```python
from build123d import *

# Parameters (mm, degrees)
SKETCH1_W           = 3.375
SKETCH1_H           = 1
CUT_EXTRUDE1_DEPTH  = 17.505188578
CIRPATTERN1_COUNT   = 3
SKETCH5_R           = 0.4
BOSS_EXTRUDE1_DEPTH = 2.5


with BuildPart() as part:
    # Sketch1 → Revolve1 (revolve)
    with BuildSketch(Plane(origin=(0, 0, 0), x_dir=(0, 0, -1), z_dir=(1, 0, 0)), mode=Mode.PRIVATE) as revolve1_sk:
        with Locations((1.6875, 15.3)):
            Rectangle(SKETCH1_W, SKETCH1_H)
    revolve(revolve1_sk.sketch.rotate(Axis((0, 33.37320456, 0), (0, -1, 0)), 180), axis=Axis((0, 33.37320456, 0), (0, -1, 0)))

    # Sketch2 → Cut-Extrude1 (cut, through all)
    with BuildSketch(Plane(origin=(0, 0, 0), x_dir=(0, 0, -1), z_dir=(1, 0, 0))):
        with BuildLine():
            Line((-0.5, 15.8), (0.5, 15.8))
            ThreePointArc((0.5, 15.8), (0.321027237, 15.781039562), (0.15, 15.725))
            Line((0.15, 15.725), (0.15, 15.65))
            Line((0.15, 15.65), (-0.15, 15.65))
            Line((-0.15, 15.65), (-0.15, 15.725))
            ThreePointArc((-0.15, 15.725), (-0.321027237, 15.781039562), (-0.5, 15.8))
        make_face()
    cut_extrude1 = extrude(amount=-CUT_EXTRUDE1_DEPTH, mode=Mode.SUBTRACT)

    # CirPattern1: Cut-Extrude1 ×3 about axis
    cirpattern1_axis = Axis((0, 0, 0), (0, 1, 0))
    for i in range(1, CIRPATTERN1_COUNT):
        add(cut_extrude1.rotate(cirpattern1_axis, i * 360 / CIRPATTERN1_COUNT), mode=Mode.SUBTRACT)

    # Sketch1_3 → Revolve2 (revolve)
    with BuildSketch(Plane(origin=(0, 0, 0), x_dir=(0, 0, -1), z_dir=(1, 0, 0)), mode=Mode.PRIVATE) as revolve2_sk:
        with BuildLine():
            Line((3.375, 15.9), (3.375, 15.8))
            Line((3.375, 15.8), (3.375, 14.8))
            Line((3.375, 14.8), (0, 14.8))
            Line((0, 14.8), (0, 0))
            Line((0, 0), (4, 0))
            Line((4, 0), (4, -0.1))
            Line((4, -0.1), (4.15, -0.1))
            ThreePointArc((4.15, -0.1), (4.857106781, 0.192893219), (5.15, 0.9))
            Line((5.15, 0.9), (5.15, 1.95))
            ThreePointArc((5.15, 1.95), (5.092538314, 2.341511494), (4.925, 2.7))
            ThreePointArc((4.925, 2.7), (4.7, 3.45), (4.925, 4.2))
            ThreePointArc((4.925, 4.2), (5.092538314, 4.558488506), (5.15, 4.95))
            Line((5.15, 4.95), (5.15, 14.9))
            ThreePointArc((5.15, 14.9), (4.857106781, 15.607106781), (4.15, 15.9))
            Line((4.15, 15.9), (3.375, 15.9))
        make_face()
    revolve(revolve2_sk.sketch.rotate(Axis((0, 33.37320456, 0), (0, -1, 0)), 180), axis=Axis((0, 33.37320456, 0), (0, -1, 0)))

    # Sketch5 → Boss-Extrude1 (add)
    with BuildSketch(Plane.XZ):
        with Locations(Location((0, 2.5, 0), (0, 0, 270))):
            Circle(SKETCH5_R)
        with Locations(Location((0, -2.5, 0), (0, 0, 90))):
            Circle(SKETCH5_R)
    extrude(amount=BOSS_EXTRUDE1_DEPTH)


solid = part.part
```
Geometry check sheet. Reference: the model listing, model coordinates, mm. A direction names the side the tool comes from. Coordinates: 2 decimals unless noted, no trailing zeros. Order: outer loops, then holes, each group sorted by start corner. A loop starts at its lowest first (then second) coordinate and runs counter-clockwise, first axis right, second up.
Item 1: Scan lines: line 1 along Y through (x, z) = (0, -1.5); line 2 along Y through (x, z) = (0.75, 1.5); line 3 along Y through (x, z) = (-4.5, 2). Record each from-to range of solid material in increasing order.
Item 2: Depth check by flat-ended pin: pin 1 (1.5 mm diameter, centred on x = 1.5, y = 1.5, fed in from -Z); pin 2 (4 mm diameter, centred on y = 0.5, z = -4, fed in from -X); pin 3 (2.5 mm diameter, centred on x = -1.5, z = 1, fed in from -Y). Enter the tip coordinate at first touch or a pass-through.
Item 3: Tool access check on faces 1 (the flat face through (0, 0, 0)), 2 (the flat face through (0, 15.65, 0)), 3 (the flat face through (2, 15.9, 3)). Record the directions out of +Z, -Z, +X, -X, +Y, -Y that give a thin tool (end or side, any length) a straight path to the whole face; none if there is none.
Item 4: Section check A-A (y = 11.5). Enter the section's corners in (x, z).
Check sheet entries:
1. line 1: y = 0 to 15.8
1. line 2: y = 0 to 15.65
1. line 3: y = 0.27 to 2.7, 4.2 to 15.53
2. pin 1: stops at z = -5.1
2. pin 2: stops at x = -4.73
2. pin 3: stops at y = 0
3. face 1: -Y
3. face 2: +Y
3. face 3: +Z, -Z, +X, -X, +Y
4. outline: circle Ø10.3 at (0, 0)
